Here's how the part is built. I have some questions about the finished solid (model axes, mm). A direction names the side the tool comes from. Round coordinates to 2 decimals unless told otherwise and drop trailing zeros. Loops run counter-clockwise (first coordinate to the right, second up) from the corner with the lowest first, then second, coordinate; pieces in that order, holes last. Notation, with made-up numbers: M 84.25,82.25 L 104.25,82.25 A14 ccw 104.25,90.25 Z; hole C 63.25,14.5 d3. An arc over 180 degrees is marked long. Answer as a JSON object with one key per item and string values.
from build123d import *

# Parameters (mm, degrees)
BOSS_EXTRUDE1_DEPTH = 7
SKETCH2_R           = 3
BOSS_EXTRUDE2_DEPTH = 1
SKETCH3_R           = 3.5
CUT_EXTRUDE1_DEPTH  = 5
SKETCH4_R           = 1.5
CUT_EXTRUDE2_DEPTH  = 32.717503054
SKETCH17_W          = 20
SKETCH17_H          = 18
BOSS_EXTRUDE6_DEPTH = 10
SKETCH18_W          = 20
SKETCH18_H          = 10
BOSS_EXTRUDE7_DEPTH = 45
CUT_EXTRUDE6_REACH  = 66.343
SKETCH19_R          = 5
FILLET4_R           = 5
FILLET6_R           = 5
FILLET8_R           = 5


with BuildPart() as part:
    # Sketch1 → Boss-Extrude1 (new body)
    with BuildSketch(Plane(origin=(0, 0, 0), x_dir=(1, 0, 0), z_dir=(0, 1, 0))):
        with BuildLine():
            Line((-21, 9), (21, 9))
            ThreePointArc((21, 9), (30, 0), (21, -9))
            Line((21, -9), (-21, -9))
            ThreePointArc((-21, -9), (-30, 0), (-21, 9))
        make_face()
    extrude(amount=BOSS_EXTRUDE1_DEPTH)

    # Sketch2 → Boss-Extrude2 (add)
    with BuildSketch(Plane.XZ):
        with Locations(Location((-21, 0, 0), (0, 0, 270))):
            Circle(SKETCH2_R)
    boss_extrude2 = extrude(amount=BOSS_EXTRUDE2_DEPTH)

    # Sketch3 → Cut-Extrude1 (cut)
    with BuildSketch(Plane(origin=(0, 7, 0), x_dir=(1, 0, 0), z_dir=(0, 1, 0))):
        with Locations(Location((-21, 0, 0), (0, 0, 270))):
            Circle(SKETCH3_R)
    cut_extrude1 = extrude(amount=-CUT_EXTRUDE1_DEPTH, mode=Mode.SUBTRACT)

    # Sketch4 → Cut-Extrude2 (cut, through all)
    with BuildSketch(Plane(origin=(0, 2, 0), x_dir=(1, 0, 0), z_dir=(0, 1, 0))):
        with Locations(Location((-21, 0, 0), (0, 0, 270))):
            Circle(SKETCH4_R)
    cut_extrude2 = extrude(amount=-CUT_EXTRUDE2_DEPTH, mode=Mode.SUBTRACT)

    # Mirror1: Boss-Extrude2, Cut-Extrude1, Cut-Extrude2 across plane
    add(boss_extrude2.mirror(Plane(origin=(0, 0, 0), x_dir=(0, 0, 1), z_dir=(1, 0, 0))))
    add(cut_extrude1.mirror(Plane(origin=(0, 0, 0), x_dir=(0, 0, 1), z_dir=(1, 0, 0))), mode=Mode.SUBTRACT)
    add(cut_extrude2.mirror(Plane(origin=(0, 0, 0), x_dir=(0, 0, 1), z_dir=(1, 0, 0))), mode=Mode.SUBTRACT)

    # Sketch17 → Boss-Extrude6 (add)
    with BuildSketch(Plane(origin=(0, 7, 0), x_dir=(1, 0, 0), z_dir=(0, 1, 0))):
        Rectangle(SKETCH17_W, SKETCH17_H)
    extrude(amount=BOSS_EXTRUDE6_DEPTH)

    # Sketch18 → Boss-Extrude7 (add)
    with BuildSketch(Plane.XY.offset(9)):
        with Locations((0, 12)):
            Rectangle(SKETCH18_W, SKETCH18_H)
    boss_extrude7 = extrude(amount=BOSS_EXTRUDE7_DEPTH)

    # Mirror3: Boss-Extrude7 across plane
    add(boss_extrude7.mirror(Plane.XY))

    # Sketch19 → Cut-Extrude6 (cut, up to next)
    with BuildSketch(Plane(origin=(0, 17, 0), x_dir=(1, 0, 0), z_dir=(0, 1, 0)), mode=Mode.PRIVATE) as cut_extrude6_sk1:
        with Locations(Location((0, 40, 0), (0, 0, 270))):
            Circle(SKETCH19_R)
    cut_extrude6_tool1 = extrude(cut_extrude6_sk1.sketch, amount=-CUT_EXTRUDE6_REACH, mode=Mode.PRIVATE) & part.part
    cut_extrude6 = cut_extrude6_tool1.solids().sort_by_distance((0, 17, -40))[0]
    add(cut_extrude6, mode=Mode.SUBTRACT)

    # Mirror4: Cut-Extrude6 across plane
    add(cut_extrude6.mirror(Plane.XY), mode=Mode.SUBTRACT)

    # Fillet4
    fillet4_edges = [part.edges().sort_by_distance(p)[0] for p in [
        (10, 7, 0),
    ]]
    fillet(fillet4_edges, radius=FILLET4_R)

    # Fillet6
    fillet6_edges = [part.edges().sort_by_distance(p)[0] for p in [
        (-10, 7, 0),
    ]]
    fillet(fillet6_edges, radius=FILLET6_R)

    # Fillet8
    fillet8_edges = [part.edges().sort_by_distance(p)[0] for p in [
        (-10, 9.5, 9),
        (-10, 9.5, -9),
        (10, 9.5, -9),
        (10, 9.5, 9),
    ]]
    fillet(fillet8_edges, radius=FILLET8_R - 0.0001)  # a hair under: the kernel refuses the full size


solid = part.part
Item 1: I want a section at A-A on z = 0. Count the separate pieces of the cut face and the enclosed holes in it, plus the area to 3 significant figures.
Solution:
{"separate pieces": "3", "enclosed holes": "0", "area": "555 mm2"}
Item 2: I want a section at C-C on z = 40. List the corners of the cut face in (x, y) for me.
Solution:
{"outline": "M -10,7 L -5,7 L -5,17 L -10,17 Z; M 5,7 L 10,7 L 10,17 L 5,17 Z"}
Item 3: For faces 5 (the face through (-23.93, -0.49, 0.65)), 6 (the face through (-17.53, 4.54, -0.46)), 7 (the face through (10, 13, 1)), 8 (the face through (-10, 13, 1)), which set-ups out of +Z, -Z, +X, -X, +Y, -Y let a thin tool reach every point of the face, with its end or its side?
Solution:
{"face 5": "-Y", "face 6": "+Y", "face 7": "+X, +Y", "face 8": "-X, +Y"}
Item 4: For P1, Ø2, axis at x = 13.5, y = 3.5, coming from the +Z side; P2, Ø10, axis at y = 6.5, z = -14.5, coming from the -X side; P3, Ø4, axis at x = -21, z = 0, coming from the +Y side; P4, Ø8, axis at y = 2, z = 34.5, coming from the +X side, each with a flat end and sliding along its axis, tell me the tip position at first contact or that it passes through.
Solution:
{"P1": "stops at z = 9", "P2": "stops at x = -12.77", "P3": "stops at y = 2", "P4": "passes through"}
Item 5: We'd pull the mould along X, two halves only. Please class faces 1 (the face through (0, 12, 54)), 2 (the face through (-19.735, 0.521, 0.806)), 3 (the face through (-10.49, 8.42, -11.84)), 4 (the face through (21, 2, 2)): +X half, -X half, draft (parallel to the pull), parting line (faces both ways), or undercut.
Solution:
{"face 1": "draft", "face 2": "undercut", "face 3": "-X half", "face 4": "undercut"}
Item 6: I want a section at B-B on x = 2. List the corners of the cut face in (y, z) for me, plus the area to 3 significant figures.
Solution:
{"outline": "M 0,-9 L 7,-9 L 7,-35.42 L 17,-35.42 L 17,35.42 L 7,35.42 L 7,9 L 0,9 Z; M 7,-54 L 17,-54 L 17,-44.58 L 7,-44.58 Z; M 7,44.58 L 17,44.58 L 17,54 L 7,54 Z", "area": "1,020 mm2"}
Item 7: I want a section at D-D on z = -11.5. List the corners of the cut face in (x, y) for me, plus the area to 3 significant figures.
Solution:
{"outline": "M -10.67,7 L 10.67,7 L 10.67,9.5 A5 cw 10,12 L 10,17 L -10,17 L -10,12 A5 cw -10.67,9.5 Z", "area": "204 mm2"}
Item 8: If I drill on L1, parallel to X at y = 5.2, z = 0; L2, parallel to X at y = 0.7, z = 0; L3, parallel to X at y = 14.5, z = 40, over which ranges is the centre line in solid material (lowest first)? Write a range as from..to.
Solution:
{"L1": "x = -30..-24.5, -17.5..17.5, 24.5..30", "L2": "x = -30..-22.5, -19.5..19.5, 22.5..30", "L3": "x = -10..-5, 5..10"}
